Model file for the job. Use its own axes, mm. A direction names the side the tool comes from. Round coordinates to 2 decimals unless told otherwise and drop trailing zeros. Order: outer loops, then holes, each group sorted by start corner. A loop starts at its lowest first (then second) coordinate and runs counter-clockwise, first axis right, second up. Notation, with made-up numbers: (-2, 46) - (22, 46) arc R31 ccw to (22, 70) - close; hole circle Ø5 at (86, 48.5). An arc over 180 degrees is marked (long way). Put each result on its own line as item: value. Start each with the question number.
Item 1: Pin check, flat tips, straight feed: pin 1 Ø4 at (x, y) = (4, -4) entering from +Z; pin 2 Ø6.5 at (x, y) = (20, -61.725) entering from -Z; pin 3 Ø3 at (y, z) = (-27.5, 39) entering from -X. Stop position of each tip, or through.
Item 2: Which spindle directions (+Z, -Z, +X, -X, +Y, -Y) get a long thin tool onto all of the face, cutting with end or side? Do faces 1 (the face through (9.5, -61.8, 2.5)), 2 (the face through (61, 0, 3)), 3 (the face through (80, -42, 32)). Say none if no direction does.
Item 3: Saw through at A-A on x = 13.5. List the corners of the cut face in (y, z) (3 decimals), plus the area to 4 significant figures.
Item 4: Saw through at B-B on y = -78.3. List the corners of the cut face in (x, z).
Item 5: Saw through at D-D on y = -4. List the corners of the cut face in (x, z).
Item 6: Probe probe 1 along Y at (x, z) = (4, 3.45); probe 2 along Y at (x, z) = (20, 3) (3 decimals); probe 3 along Z at (x, y) = (65.5, -40). List the from-to ranges inside material, lowest first.
Item 7: Saw through at C-C on z = 56. List the corners of the cut face in (x, y).
Item 8: Mould opens along Z. For faces 4 (the face through (82, -41, 60)), 5 (the face through (42, -41, 0)), 6 (the face through (82.535, -77.185, 57.216)), 7 (the face through (14, -63.725, 3)) say: pulls with the +Z half, pulls with the -Z half, needs draft (parallel to the pull), parting line crosses it, or undercut.
```python
from build123d import *

# Parameters (mm, degrees)
SKETCH1_W            = 85
SKETCH1_H            = 82.3
BOSS_EXTRUDE1_DEPTH  = 60
SKETCH2_W            = 80
SKETCH2_H            = 55
CUT_EXTRUDE1_DEPTH   = 83.3
CUT_EXTRUDE2_DEPTH   = 50
FILLET1_R            = 0.5
FILLET1_OF_MIRROR1_R = 0.5
SKETCH4_R            = 1.65
CUT_EXTRUDE3_DEPTH   = 20
SKETCH5_R            = 1.65
CUT_EXTRUDE4_DEPTH   = 20


with BuildPart() as part:
    # Sketch1 → Boss-Extrude1 (new body)
    with BuildSketch(Plane.XY):
        with Locations((42.5, -41.15)):
            Rectangle(SKETCH1_W, SKETCH1_H)
    extrude(amount=BOSS_EXTRUDE1_DEPTH)

    # Sketch2 → Cut-Extrude1 (cut, through all)
    with BuildSketch(Plane.XZ.offset(82.3)):
        with Locations((40, 32.5)):
            Rectangle(SKETCH2_W, SKETCH2_H)
    extrude(amount=-CUT_EXTRUDE1_DEPTH, mode=Mode.SUBTRACT)

    # Sketch3 → Cut-Extrude2 (cut)
    with BuildSketch(Plane.XY.offset(5)):
        with BuildLine():
            Line((16.535898385, -63.725), (11.5, -63.725))
            ThreePointArc((11.5, -63.725), (9.5, -61.725), (11.5, -59.725))
            Line((11.5, -59.725), (16.535898385, -59.725))
            ThreePointArc((16.535898385, -59.725), (24, -61.725), (16.535898385, -63.725))
        make_face()
    cut_extrude2 = extrude(amount=-CUT_EXTRUDE2_DEPTH, mode=Mode.SUBTRACT)

    # Fillet1
    fillet1_edges = [part.edges().sort_by_distance(p)[0] for p in [
        (16.535898385, -59.725, 2.5),
        (16.535898385, -63.725, 2.5),
    ]]
    fillet(fillet1_edges, radius=FILLET1_R)

    # Mirror1: Cut-Extrude2 across plane
    add(cut_extrude2.mirror(Plane(origin=(0, -41.15, 0), x_dir=(0, 0, 1), z_dir=(0, -1, 0))), mode=Mode.SUBTRACT)

    # Fillet1 of Mirror1
    fillet1_of_mirror1_edges = [part.edges().sort_by_distance(p)[0] for p in [
        (16.535898385, -22.575, 2.5),
        (16.535898385, -18.575, 2.5),
    ]]
    fillet(fillet1_of_mirror1_edges, radius=FILLET1_OF_MIRROR1_R)

    # Sketch4 → Cut-Extrude3 (cut)
    with BuildSketch(Plane(origin=(85, 0, 0), x_dir=(0, 0, -1), z_dir=(1, 0, 0))):
        with Locations((-56, -78.3)):
            Circle(SKETCH4_R)
    extrude(amount=-CUT_EXTRUDE3_DEPTH, mode=Mode.SUBTRACT)

    # Sketch5 → Cut-Extrude4 (cut)
    with BuildSketch(Plane(origin=(0, 0, 0), x_dir=(-1, 0, 0), z_dir=(0, 0, -1))):
        with Locations((-4, -4)):
            Circle(SKETCH5_R)
        with Locations((-4, -78.3)):
            Circle(SKETCH5_R)
    extrude(amount=-CUT_EXTRUDE4_DEPTH, mode=Mode.SUBTRACT)


solid = part.part
```
Results found:
1. pin 1: stops at z = 5
1. pin 2: passes through
1. pin 3: stops at x = 80
2. face 1: +Z, -Z
2. face 2: +Z, -Z, +X, -X, +Y
2. face 3: +Z, -X, +Y, -Y
3. outline: (-82.3, 0) - (-63.725, 0) - (-63.725, 5) - (-82.3, 5) - close; (-59.725, 0) - (-22.575, 0) - (-22.575, 5) - (-59.725, 5) - close; (-18.575, 0) - (0, 0) - (0, 5) - (-18.575, 5) - close
3. area: 371.5 mm²
4. outline: (0, 0) - (2.35, 0) - (2.35, 5) - (0, 5) - close; (5.65, 0) - (85, 0) - (85, 54.35) - (80, 54.35) - (80, 5) - (5.65, 5) - close; (80, 57.65) - (85, 57.65) - (85, 60) - (80, 60) - close
5. outline: (0, 0) - (2.35, 0) - (2.35, 5) - (0, 5) - close; (5.65, 0) - (85, 0) - (85, 60) - (80, 60) - (80, 5) - (5.65, 5) - close
6. probe 1: y = -82.3 to -79.95, -76.65 to -5.65, -2.35 to 0
6. probe 2: y = -82.3 to -65.725, -57.725 to -24.575, -16.575 to 0
6. probe 3: z = 0 to 5
7. outline: (80, -82.3) - (85, -82.3) - (85, -79.95) - (80, -79.95) - close; (80, -76.65) - (85, -76.65) - (85, 0) - (80, 0) - close
8. face 4: pulls with the +Z half
8. face 5: pulls with the -Z half
8. face 6: undercut
8. face 7: needs draft
